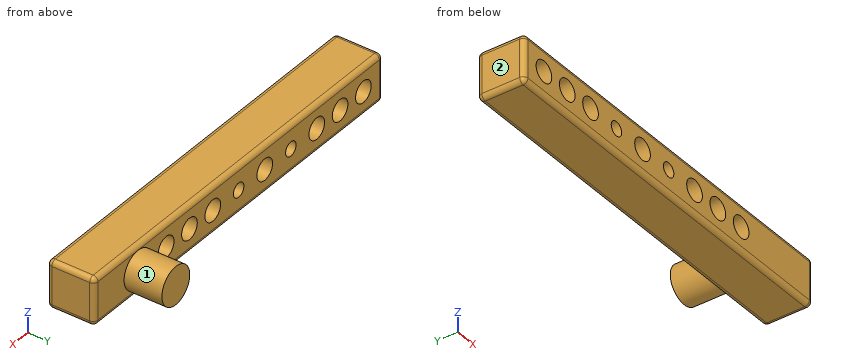
Autodesk Inventor part; units mm, degrees
ref_plane "YZ Plane" through (0, 0, 0) normal (1, 0, 0) x (0, 1, 0)
ref_plane "XZ Plane" through (0, 0, 0) normal (0, 1, 0) x (-1, 0, 0)
ref_plane "XY Plane" through (0, 0, 0) normal (0, 0, 1) x (1, 0, 0)
sketch "Sketch1" plane through (0, 0, 0) normal (0, 1, 0) x (-1, 0, 0)
  line L0 (0, 0) -> (170, 0)
  line L1 (170, 0) -> (170, 10)
  line L2 (170, 10) -> (0, 10)
  line L3 (0, 10) -> (0, 0)
  dimension "d0" = 170
  dimension "d1" = 10
extrude "Extrusion1" add sketch "Sketch1" along normal blind 10
sketch "Sketch2" plane through (0, 10, 0) normal (0, 1, 0) x (1, 0, 0)
  line L0 (0, -10) -> (0, 0)
  line L1 (0, -5) -> (-2.2, -5)
  circle A0 centre (-6.1, -5) radius 3.9
  line L2 (0, 0) -> (-170, 0)
  line L3 (-170, -10) -> (0, -10)
  circle A1 centre (-75, -5) radius 1.5
  circle A2 centre (-95, -5) radius 1.5
  dimension "d4" = 2.2
  dimension "d8" = 3
  dimension "d9" = 3
extrude "Extrusion2" cut sketch "Sketch2" against normal blind 10 contours A1
extrude "Extrusion3" cut sketch "Sketch2" against normal blind 10 contours A2
extrude "Extrusion4" cut sketch "Sketch2" against normal blind 10 contours A0
sketch "Sketch3" plane through (0, 10, 0) normal (0, 1, 0) x (1, 0, 0)
  line L0 (-170, 0) -> (-170, -10)
  line L1 (-170, -5) -> (-10, -5)
  circle A0 centre (-6.1, -5) radius 3.9
  line L2 (-165.7, -5) -> (-163.45, -5)
  circle A1 centre (-163.45, -5) radius 2.25
  circle A2 centre (-153.45, -5) radius 2.25
  circle A3 centre (-143.45, -5) radius 2.25
  circle A4 centre (-133.45, -5) radius 2.25
  circle A5 centre (-123.45, -5) radius 2.25
  circle A6 centre (-113.45, -5) radius 2.25
  circle A7 centre (-103.45, -5) radius 2.25
  circle A8 centre (-95, -5) radius 1.5
  line L3 (-93.5, -5) -> (-93.5, -7.9104)
  circle A9 centre (-75, -5) radius 1.5
  line L4 (-76.5, -5) -> (-76.5, -7.25)
  line L5 (-93.5, -5) -> (-76.5, -5)
  line L6 (-85, -5) -> (-93.5, -5)
  line L7 (-85, -5) -> (-76.5, -5)
  circle A10 centre (-80.75, -5) radius 2.25
  circle A11 centre (-89.25, -5) radius 2.25
  line L8 (-10, -5) -> (-12, -5)
  line L9 (-10, -5) -> (-14.3, -5)
  line L10 (-14.3, -5) -> (-16.55, -5)
  circle A12 centre (-16.55, -5) radius 2.25
  circle A13 centre (-26.55, -5) radius 2.25
  circle A14 centre (-36.55, -5) radius 2.25
  circle A15 centre (-46.55, -5) radius 2.25
  circle A16 centre (-56.55, -5) radius 2.25
  circle A17 centre (-66.55, -5) radius 2.25
  point P0 (0, 0)
  point P1 (-155.7, -5)
  point P2 (-145.7, -5)
  point P3 (-135.7, -5)
  point P4 (-125.7, -5)
  point P5 (-115.7, -5)
  point P6 (-105.7, -5)
  point P7 (-24.3, -5)
  point P8 (-34.3, -5)
  point P9 (-44.3, -5)
  point P10 (-54.3, -5)
  point P11 (-64.3, -5)
  dimension "d20" = 10
  dimension "d32" = 10
extrude "Extrusion5" cut sketch "Sketch3" against normal blind 10 contours A1 L1 | L1 A1 | L1 A12 | L1 A12 | A2 L1 | L1 A2 | A3 L1 | L1 A3 | A4 L1 | L1 A4 | A5 L1 | L1 A5 | A6 L1 | L1 A6 | A7 L1 | L1 A7 | A11 L1 | L1 A11 | A10 L1 | L1 A10 | A17 L1 | L1 A17 | A16 L1 | L1 A16 | A15 L1 | L1 A15 | A14 L1 | L1 A14 | A13 L1 | L1 A13
thread "Thread1"
thread "Thread2"
sketch "Sketch4" plane through (0, 10, 0) normal (0, 1, 0) x (1, 0, 0)
  circle A0 centre (-16.55, -5) radius 2.25
  circle A1 centre (-16.55, -5) radius 2.25
  point P0 (0, 0)
extrude "Extrusion6" add sketch "Sketch4" against normal blind 10
sketch "Sketch5" plane through (0, 0, 10) normal (1, 0, 0) x (0, 0, -1)
  line L0 (10, 0) -> (0, 0)
  line L1 (0, 0) -> (0, 10)
  line L2 (10, 0) -> (0, 0)
  line L3 (0, 0) -> (0, 10)
  line L4 (0, 10) -> (10, 10)
  line L5 (10, 10) -> (10, 0)
extrude "Extrusion7" add sketch "Sketch5" along normal blind 10
sketch "Sketch6" plane through (10, 0, 10) normal (1, 0, 0) x (0, 0, -1)
  line L0 (0, 0) -> (10, 0)
  line L1 (0, 10) -> (0, 0)
  line L2 (10, 0) -> (0, 0)
  line L3 (0, 0) -> (0, 10)
  line L4 (0, 10) -> (10, 10)
  line L5 (10, 10) -> (10, 0)
extrude "Extrusion8" add sketch "Sketch6" along normal blind 10
sketch "Sketch7" plane through (0, 10, 0) normal (0, 1, 0) x (1, 0, 0)
  point P0 (0, 0)
fillet "Fillet3" radius 1 11 edges at (-75, 10, 10) (-75, 0, 10) (-75, 10, 0) (20, 5, 10) (20, 5, 0) (20, 0, 5) (-170, 10, 5) (-170, 5, 10) (-170, 5, 0) (-170, 0, 5) (-75, 0, 0)
fillet "Fillet4" radius 1 3 edges at (19.7071, 9.7071, 9.7071) (19.7071, 9.7071, 0.2929) (20, 10, 5)
sketch "Sketch8" plane through (19, 1, 0) normal (0, 0, -1) x (-1, 0, 0)
  point P0 (19, -1)
sketch "Sketch9" plane through (0, 10, 0) normal (0, 1, 0) x (1, 0, 0)
  circle A0 centre (-6.1, -5) radius 3.9
  circle A1 centre (-6.1, -5) radius 2.5
  point P0 (0, 0)
  dimension "d53" = 5
extrude "Extrusion9" add sketch "Sketch9" against normal blind 10
sketch "Sketch10" plane through (0, 10, 0) normal (0, 1, 0) x (1, 0, 0)
  circle A0 centre (-6.1, -5) radius 2.5
  line L0 (-3.6, -5) -> (1.4, -5)
  line L1 (19, -9) -> (19, -1)
  line L2 (1.4, -5) -> (-76.5, -5)
  circle A1 centre (-75, -5) radius 1.5
  line L3 (-76.5, -5) -> (-76.5, -10.0231)
  line L4 (-76.5, -10.0231) -> (-76.5, 0)
  line L5 (-76.5, -10.0231) -> (-169.9715, -10.0231)
  line L6 (-169, -9) -> (19, -9)
  line L7 (-169.9715, 0) -> (-76.5, 0)
  line L8 (-169.9715, -10.0231) -> (-170.1763, -9.372)
  line L9 (-170.1763, -9.372) -> (-170.4489, -3.7164)
  line L10 (-170.4489, -3.7164) -> (-170.4593, -3.5)
  line L11 (-170.4593, -3.5) -> (-170.4593, -0.543)
  line L12 (-170.4593, -0.543) -> (-169.9715, 0)
  point P0 (0, 0)
  dimension "d56" = 5
extrude "Extrusion10" cut sketch "Sketch10" against normal blind 10 contours L3 L5 L8 L9 L10 L11 L12 L7 L4
sketch "Sketch11" plane through (0, 10, 0) normal (0, 1, 0) x (1, 0, 0)
  circle A0 centre (-75, -5) radius 1.5
  circle A1 centre (-75, -5) radius 1.5
  circle A2 centre (-66.55, -5) radius 2.25
  circle A3 centre (-66.55, -5) radius 2.25
  circle A4 centre (-56.55, -5) radius 2.25
  circle A5 centre (-56.55, -5) radius 2.25
  circle A6 centre (-46.55, -5) radius 2.25
  circle A7 centre (-46.55, -5) radius 2.25
  circle A8 centre (-36.55, -5) radius 2.25
  circle A9 centre (-36.55, -5) radius 2.25
  circle A10 centre (-26.55, -5) radius 2.25
  circle A11 centre (-26.55, -5) radius 2.25
  point P0 (0, 0)
  point P1 (-76.5, -5)
extrude "Extrusion11" add sketch "Sketch11" against normal blind 10
sketch "Sketch12" plane through (0, 10, 0) normal (0, 1, 0) x (1, 0, 0)
  circle A0 centre (-6.1, -5) radius 2.5
  line L0 (-8.6, -5) -> (-76.5, -5)
  line L1 (-76.5, -9) -> (-76.5, -1)
  line L2 (-42.55, -5) -> (-27.55, -5)
  line L3 (-42.55, -5) -> (-57.55, -5)
  line L4 (-42.55, -5) -> (-50.05, -5)
  line L5 (-42.55, -5) -> (-35.05, -5)
  circle A1 centre (-50.05, -5) radius 1.5
  circle A2 centre (-35.05, -5) radius 1.5
  line L6 (-3.6, -5) -> (6.4143, -5)
  line L7 (6.4143, -5) -> (6.4143, -10.3738)
  line L8 (6.4143, -10.3738) -> (6.4143, 1.3096)
  line L9 (6.4143, 1.3096) -> (23.7189, 1.3096)
  line L10 (23.7189, 1.3096) -> (24.3802, -13.5702)
  line L11 (24.3802, -13.5702) -> (6.4143, -10.3738)
  point P0 (0, 0)
  dimension "d61" = 15
  dimension "d62" = 15
  dimension "d63" = 3
  dimension "d64" = 3
extrude "Extrusion12" cut sketch "Sketch12" against normal blind 10 contours A2 L0 | L0 A2 | A1 L0 | L0 A1 | L8 L9 L10 L11 L7
sketch "Sketch13" plane through (0, 10, 0) normal (0, 1, 0) x (1, 0, 0)
  circle A0 centre (-50.05, -5) radius 1.5
  line L0 (-48.55, -5) -> (-36.55, -5)
  circle A1 centre (-35.05, -5) radius 1.5
  circle A2 centre (-42.55, -5) radius 2.25
  line L1 (-51.55, -5) -> (-55.25, -5)
  line L2 (-33.55, -5) -> (-29.85, -5)
  circle A3 centre (-57.5, -5) radius 2.25
  circle A4 centre (-27.6, -5) radius 2.25
  circle A5 centre (-20.9, -5) radius 2.25
  circle A6 centre (-14.2, -5) radius 2.25
  circle A7 centre (-64.2, -5) radius 2.25
  circle A8 centre (-70.9, -5) radius 2.25
  point P0 (0, 0)
  dimension "d67" = 4.5
  dimension "d68" = 3.7
  dimension "d69" = 3.7
  dimension "d71" = 4.5
  dimension "d73" = 4.5
  dimension "d83" = 6.7
  dimension "d90" = 6.7
extrude "Extrusion13" cut sketch "Sketch13" against normal blind 10 contours A3 | A4 | A5 | A6 | A7 | A8
sketch "Sketch14" plane through (0, 10, 0) normal (0, 1, 0) x (1, 0, 0)
  circle A0 centre (-57.5, -5) radius 2.25
  line L0 (-55.25, -5) -> (-29.85, -5)
  circle A1 centre (-27.6, -5) radius 2.25
  circle A2 centre (-42.55, -5) radius 2.25
  point P0 (0, 0)
  dimension "d97" = 4.5
extrude "Extrusion14" cut sketch "Sketch14" against normal blind 10 contours A2 L0 | L0 A2
thread "Thread3"
thread "Thread4"
fillet "Fillet5" radius 1 16 edges at (-76.5, 9.7071, 9.7071) (-76.5, 5, 10) (-76.5, 0.2929, 9.7071) (-76.5, 0, 5) (-76.5, 0.2929, 0.2929) (-76.5, 5, 0) (-76.5, 9.7071, 0.2929) (-76.5, 10, 5) (6.4143, 9.7071, 0.2929) (6.4143, 5, 0) (6.4143, 0.2929, 0.2929) (6.4143, 0, 5) (6.4143, 0.2929, 9.7071) (6.4143, 5, 10) (6.4143, 9.7071, 9.7071) (6.4143, 10, 5)
sketch "Sketch15" plane through (0, 10, 0) normal (0, 1, 0) x (1, 0, 0)
  circle A0 centre (-6.1, -5) radius 2.5
  circle A1 centre (-6.1, -5) radius 2.75
  point P0 (0, 0)
  dimension "d105" = 5.5
extrude "Extrusion15" cut sketch "Sketch15" against normal blind 10 contours A0 | A1
sketch "Sketch16" plane through (0, 10, 0) normal (0, 1, 0) x (1, 0, 0)
  circle A0 centre (-6.1, -5) radius 2.75
  circle A1 centre (-6.1, -5) radius 4
  point P0 (0, 0)
  dimension "d108" = 8
extrude "Extrusion16" add sketch "Sketch16" against normal blind 10 contours A0 | A1
extrude "Extrusion17" add sketch "Sketch16" along normal blind 8 contours A0 | A1
properties part number "brazo de servo el d vdd - camara"
Model file for the job. Use its own axes, mm. Face numbers are marked on the shaded views. A direction names the side the tool comes from. Give positions to 0.01 mm unless a question says otherwise; leave off trailing zeros. Order: outer loops, then holes, each group sorted by start corner. A loop starts at its lowest first (then second) coordinate and runs counter-clockwise, first axis right, second up. Notation, with made-up numbers: M -9,29 L 35,29 A15 ccw 35,39 Z; hole C -18.75,42.25 d4. An arc over 180 degrees is marked long. Put each result on its own line as item: value. Start each with the question number.
(1) Band-saw the part on C-C on x = -31.5. Give the cut face in (y, z), then the cut area to 3 significant figures.
(2) Band-saw the part on D-D on x = -50.05. Give the cut face in (y, z), then the cut area to 3 significant figures.
(3) Band-saw the part on B-B on y = 6.75. Count the separate pieces of the cut face and the enclosed holes in it, then the cut area to 3 significant figures.
(4) Drill centre lines: L1, parallel to Z at x = -14.2, y = 8; L2, parallel to Y at x = -33.5, z = 8; L3, parallel to Z at x = -50.05, y = 3. Where is each one in solid material? Low to high. Write a range as [from, to].
(5) Tool access for the marked faces 1 and 2: list every direction of +Z, -Z, +X, -X, +Y, -Y with a clear straight run to the whole face (end or side of a thin tool).
(6) Band-saw the part on A-A on x = -20.9. Give the cut face in (y, z), then the cut area to 3 significant figures.
(7) Pin check, flat tip, straight feed: pin 1 Ø6 at (x, z) = (-40.5, 7.5) entering from +Y. Stop position of the tip, or through.
Results below:
1. outline: M 0,1 A1 ccw 1,0 L 9,0 A1 ccw 10,1 L 10,9 A1 ccw 9,10 L 1,10 A1 ccw 0,9 Z
1. area: 99.1 mm2
2. outline: M 0,1 A1 ccw 1,0 L 9,0 A1 ccw 10,1 L 10,3.5 L 0,3.5 Z; M 0,6.5 L 10,6.5 L 10,9 A1 ccw 9,10 L 1,10 A1 ccw 0,9 Z
2. area: 69.1 mm2
3. separate pieces: 1
3. enclosed holes: 9
3. area: 703 mm2
4. L1: z = [0, 2.75], [7.25, 10]
4. L2: y = [0, 10]
4. L3: z = [0, 3.5], [6.5, 10]
5. face 1: +Y
5. face 2: +Z, -Z, -X, +Y, -Y
6. outline: M 0,1 A1 ccw 1,0 L 9,0 A1 ccw 10,1 L 10,2.75 L 0,2.75 Z; M 0,7.25 L 10,7.25 L 10,9 A1 ccw 9,10 L 1,10 A1 ccw 0,9 Z
6. area: 54.1 mm2
7. pin 1: stops at y = 10
